Work out the finished part from the listing and answer in its coordinate system (mm). A direction names the side the tool comes from. Coordinates: 2 decimals unless noted, no trailing zeros. Loops run counter-clockwise (first coordinate to the right, second up) from the corner with the lowest first, then second, coordinate; pieces in that order, holes last. Notation, with made-up numbers: (51, 53.5) - (70, 53.5) arc R20 ccw to (70, 69.5) - close; hole circle Ø2 at (9, 85.25). An arc over 180 degrees is marked (long way). Write each question's results on one line, items separated by ' | '. Start each with the question number.
1. A cutting plane is placed at C-C on x = 6.5. Determine the outline of the cut face in (y, z) (3 decimals).
2. Determine the mould class of faces 3 (the flat face through (16, 13, 0)), 4 (the flat face through (13, 25.4, 1)), 5 (the cylindrical face through (0.966, 11.377, 24.044)), 6 (the flat face through (32, 13, 25.4)) for opening direction Z: released by +Z, released by -Z, zero draft, split by the parting line, or undercut.
3. Which of the six approach directions +Z, -Z, +X, -X, +Y, -Y give full straight-line access (tool end or side, diameter ignored) to faces 1 (the flat face through (31.115, 4, 8)), 2 (the flat face through (33.02, 10, 4))?
4. A cutting plane is placed at B-B on z = 13.97. Determine the outline of the cut face in (x, y) (3 decimals), then the cut area to 3 significant figures.
5. This flat-tipped pin is pushed along its axis until it touches: P1, Ø12, axis at y = 12.7, z = 13.97, coming from the -X side. Where does it stop, or does it pass through?
6. Find the intervals of material crossed by line 1 along X through (y, z) = (2.25, 4.5) (3 decimals); line 2 along Z through (x, y) = (0.85, 12.7); line 3 along Z through (x, y) = (23.5, 15.75) (3 decimals), in increasing order. Write a range as [from, to].
7. A cutting plane is placed at D-D on z = 9.25. Determine the outline of the cut face in (x, y) (3 decimals), then the cut area to 3 significant figures.
8. A cutting plane is placed at A-A on y = 12.7. Determine the outline of the cut face in (x, z) (3 decimals).
from build123d import *

# Parameters (mm, degrees)
F0_W     = 33.02
F0_H     = 25.4
F1_DEPTH = 25.4
F2_R     = 10.16
F3_DEPTH = 50.8
F4_W     = 29.21
F4_H     = 23.495
F5_DEPTH = 25.4


with BuildPart() as f1:
    # F0 (on Top) → F1 (new body)
    with BuildSketch(Plane.XY):
        with Locations((16.51, 12.7)):
            Rectangle(F0_W, F0_H)
    extrude(amount=F1_DEPTH)

    # F2 (on face) → F3 (cut)
    with BuildSketch(Plane.YZ.offset(33.02)):
        with Locations((12.7, 13.97)):
            Circle(F2_R)
    extrude(amount=-F3_DEPTH, mode=Mode.SUBTRACT)

    # F4 (on face) → F5 (cut)
    with BuildSketch(Plane.XZ):
        with Locations((16.51, 13.6525)):
            Rectangle(F4_W, F4_H)
    extrude(amount=-F5_DEPTH, mode=Mode.SUBTRACT)


solid = f1.part
Values:
1) outline: (0, 0) - (25.4, 0) - (25.4, 1.905) - (0, 1.905) - close
2) face 3: released by -Z | face 4: zero draft | face 5: undercut | face 6: released by +Z
3) face 1: +Z, +Y, -Y | face 2: +Z, -Z, +X, +Y, -Y
4) outline: (0, 0) - (1.905, 0) - (1.905, 2.54) - (0, 2.54) - close; (0, 22.86) - (1.905, 22.86) - (1.905, 25.4) - (0, 25.4) - close; (31.115, 0) - (33.02, 0) - (33.02, 2.54) - (31.115, 2.54) - close; (31.115, 22.86) - (33.02, 22.86) - (33.02, 25.4) - (31.115, 25.4) - close | area: 19.4 mm^2
5) P1: through
6) line 1: [0, 1.905], [31.115, 33.02] | line 2: [0, 3.81], [24.13, 25.4] | line 3: [0, 1.905]
7) outline: (0, 0) - (1.905, 0) - (1.905, 3.703) - (0, 3.703) - close; (0, 21.697) - (1.905, 21.697) - (1.905, 25.4) - (0, 25.4) - close; (31.115, 0) - (33.02, 0) - (33.02, 3.703) - (31.115, 3.703) - close; (31.115, 21.697) - (33.02, 21.697) - (33.02, 25.4) - (31.115, 25.4) - close | area: 28.2 mm^2
8) outline: (0, 0) - (33.02, 0) - (33.02, 3.81) - (31.115, 3.81) - (31.115, 1.905) - (1.905, 1.905) - (1.905, 3.81) - (0, 3.81) - close; (0, 24.13) - (1.905, 24.13) - (1.905, 25.4) - (0, 25.4) - close; (31.115, 24.13) - (33.02, 24.13) - (33.02, 25.4) - (31.115, 25.4) - close
